Design review of the part built by this model. Coordinates are the model's own, in mm. Face numbers are marked on the shaded views. A direction names the side the tool comes from. Coordinates: 2 decimals unless noted, no trailing zeros. Loops run counter-clockwise (first coordinate to the right, second up) from the corner with the lowest first, then second, coordinate; pieces in that order, holes last. Notation, with made-up numbers: (54, 38) - (88, 38) arc R20 ccw to (88, 57) - close; hole circle Ø8 at (-0.75, -28). An arc over 180 degrees is marked (long way). Use one line per item in the form item = value. Start each with the question number.
(1) Clearance check with flat-ended pins moving along their axes: pin 1 Ø6 at (x, z) = (18, 10.5) entering from -Y; pin 2 Ø1.2 at (x, y) = (-1.5, 7.5) entering from +Z; pin 3 Ø2 at (x, y) = (15, 22) entering from +Z; pin 4 Ø2 at (x, z) = (-34, 3) entering from -Y. State where each tip first meets the part, or that it passes through.
(2) For L1, parallel to Z at x = 34, y = 3; L2, parallel to Z at x = 34, y = 8.75; L3, parallel to Y at x = 0, z = 1.15, list the stretches that pass through material, from the lowest coordinate up.
(3) Add section A-A (z = 3). State the section outline as (x, y) points, plus the area to 3 significant figures.
(4) Tool access review of the marked faces 5, 6 and 7: name each direction out of +Z, -Z, +X, -X, +Y, -Y from which nothing blocks a thin tool from reaching the whole face with its end or side.
(5) Add section D-D (x = 1). State the section outline as (y, z) points.
(6) Add section B-B (x = -28). State the section outline as (y, z) points.
(7) Add section C-C (y = 21.5). State the section outline as (x, z) points.
(8) The part is to be moulded in two halves that separate along Y. For the marked faces 1, 2, 3 and 4, say which applies: pulls with the +Y half, pulls with the -Y half, needs draft (parallel to the pull), parting line crosses it, or undercut.
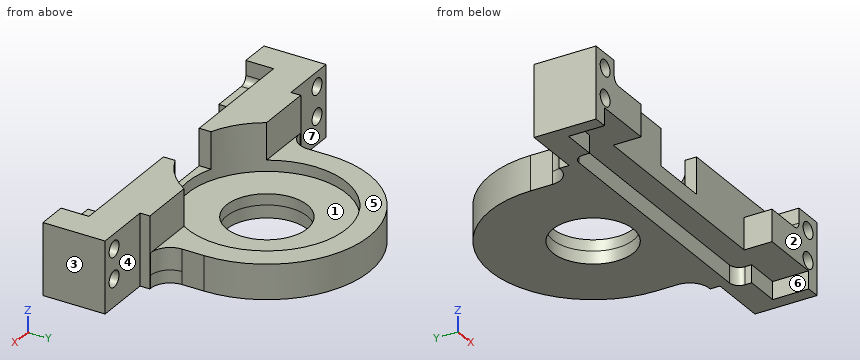
```python
from build123d import *

# Parameters (mm, degrees)
SKETCH2_R           = 16
BOSS_EXTRUDE1_DEPTH = 12
SKETCH3_R           = 16
SKETCH3_R_2         = 8.25
BOSS_EXTRUDE2_DEPTH = 2.5
CUT_EXTRUDE4_DEPTH  = 1
CUT_EXTRUDE5_REACH  = 60.683
SKETCH9_W           = 43.9
SKETCH9_H           = 5.7
SKETCH10_R          = 1.65
CUT_EXTRUDE6_DEPTH  = 59.87817932
CUT_EXTRUDE7_START  = -7.5
CUT_EXTRUDE7_DEPTH  = 7.5
FILETE1_R           = 2
FILETE2_R           = 4
SKETCH12_W          = 9
SKETCH12_H          = 5.7
CUT_EXTRUDE8_DEPTH  = 4.5
SKETCH15_W          = 12
SKETCH15_H          = 2.667603026
CUT_EXTRUDE10_DEPTH = 7.5
SKETCH16_R          = 8.25
BOSS_EXTRUDE3_DEPTH = 2.6
FILLET2_R           = 1.5
CUT_EXTRUDE11_REACH = 61.463
SKETCH17_W          = 11.722279144
SKETCH17_H          = 2
CUT_EXTRUDE12_START = -2.25
SKETCH18_R          = 16.25
CUT_EXTRUDE12_DEPTH = 9.75


with BuildPart() as part:
    # Sketch2 → Boss-Extrude1 (new body)
    with BuildSketch(Plane.XY):
        with BuildLine():
            Line((-21, 0), (21, 0))
            Line((21, 0), (37, 0))
            Line((37, 0), (37, 14.7))
            Line((37, 14.7), (21, 14.7))
            Line((21, 14.7), (21, 23.2))
            ThreePointArc((21, 23.2), (0, 44.2), (-21, 23.2))
            Line((-21, 23.2), (-21, 14.7))
            Line((-21, 14.7), (-37, 14.7))
            Line((-37, 14.7), (-37, 0))
            Line((-37, 0), (-21, 0))
        make_face()
        with Locations((0, 23.2)):
            Circle(SKETCH2_R, mode=Mode.SUBTRACT)
    extrude(amount=BOSS_EXTRUDE1_DEPTH)

    # Sketch3 → Boss-Extrude2 (add)
    with BuildSketch(Plane.XY):
        with Locations((0, 23.2)):
            Circle(SKETCH3_R)
        with Locations((0, 23.2)):
            Circle(SKETCH3_R_2, mode=Mode.SUBTRACT)
    extrude(amount=BOSS_EXTRUDE2_DEPTH)

    # Sketch8 → Cut-Extrude4 (cut)
    with BuildSketch(Plane.XY):
        Polygon((-27.15, 0), (27.15, 0), (34.2, 0), (34.2, 7.35), (27.15, 7.35), (27.15, 10.7), (-27.15, 10.7), (-27.15, 7.35), (-34.2, 7.35), (-34.2, 0), align=None)
    extrude(amount=CUT_EXTRUDE4_DEPTH, mode=Mode.SUBTRACT)

    # Sketch9 → Cut-Extrude5 (cut, up to next)
    with BuildSketch(Plane(origin=(0, 0, 1), x_dir=(-1, 0, 0), z_dir=(0, 0, -1)), mode=Mode.PRIVATE) as cut_extrude5_sk1:
        with Locations((0, 2.85)):
            Rectangle(SKETCH9_W, SKETCH9_H)
    cut_extrude5_tool1 = extrude(cut_extrude5_sk1.sketch, amount=-CUT_EXTRUDE5_REACH, mode=Mode.PRIVATE) & part.part
    add(cut_extrude5_tool1.solids().sort_by_distance((0, 2.85, 1))[0], mode=Mode.SUBTRACT)

    # Sketch10 → Cut-Extrude6 (cut, through all)
    with BuildSketch(Plane.XZ):
        with Locations((-34, 9)):
            Circle(SKETCH10_R)
        with Locations((-34, 3)):
            Circle(SKETCH10_R)
        with Locations((34, 3)):
            Circle(SKETCH10_R)
        with Locations((34, 9)):
            Circle(SKETCH10_R)
    extrude(amount=-CUT_EXTRUDE6_DEPTH, mode=Mode.SUBTRACT)

    # Sketch11 → Cut-Extrude7 (cut)
    with BuildSketch(Plane.XY.offset(12).offset(CUT_EXTRUDE7_START)):
        with BuildLine():
            Line((21, 14.7), (21, 23.2))
            ThreePointArc((21, 23.2), (0, 44.2), (-21, 23.2))
            Line((-21, 23.2), (-21, 14.7))
            Line((-21, 14.7), (21, 14.7))
        make_face()
    extrude(amount=CUT_EXTRUDE7_DEPTH, mode=Mode.SUBTRACT)

    # Filete1
    filete1_edges = [part.edges().sort_by_distance(p)[0] for p in [
        (27.15, 10.7, 0.5),
        (-27.15, 10.7, 0.5),
    ]]
    fillet(filete1_edges, radius=FILETE1_R)

    # Filete2
    filete2_edges = [part.edges().sort_by_distance(p)[0] for p in [
        (-21, 14.7, 2.25),
        (21, 14.7, 2.25),
    ]]
    fillet(filete2_edges, radius=FILETE2_R)

    # Sketch12 → Cut-Extrude8 (cut)
    with BuildSketch(Plane.XY.offset(12)):
        with Locations((26.45, 2.85)):
            Rectangle(SKETCH12_W, SKETCH12_H)
        with Locations((-26.45, 2.85)):
            Rectangle(SKETCH12_W, SKETCH12_H)
    extrude(amount=-CUT_EXTRUDE8_DEPTH, mode=Mode.SUBTRACT)

    # Sketch15 → Cut-Extrude10 (cut)
    with BuildSketch(Plane.XY.offset(12)):
        with Locations((0, 7.033801513)):
            Rectangle(SKETCH15_W, SKETCH15_H)
    extrude(amount=-CUT_EXTRUDE10_DEPTH, mode=Mode.SUBTRACT)

    # Sketch16 → Boss-Extrude3 (add)
    with BuildSketch(Plane(origin=(0, 0, 0), x_dir=(-1, 0, 0), z_dir=(0, 0, -1))):
        with BuildLine():
            Line((-37, 14.7), (-25, 14.7))
            ThreePointArc((-25, 14.7), (-22.171572875, 15.871572875), (-21, 18.7))
            Line((-21, 18.7), (-21, 23.2))
            ThreePointArc((-21, 23.2), (0, 44.2), (21, 23.2))
            Line((21, 23.2), (21, 18.7))
            ThreePointArc((21, 18.7), (22.171572875, 15.871572875), (25, 14.7))
            Line((25, 14.7), (37, 14.7))
            Line((37, 14.7), (37, 0))
            Line((37, 0), (34.2, 0))
            Line((34.2, 0), (34.2, 7.35))
            Line((34.2, 7.35), (27.15, 7.35))
            Line((27.15, 7.35), (27.15, 8.7))
            ThreePointArc((27.15, 8.7), (26.564213562, 10.114213562), (25.15, 10.7))
            Line((25.15, 10.7), (-25.15, 10.7))
            ThreePointArc((-25.15, 10.7), (-26.564213562, 10.114213562), (-27.15, 8.7))
            Line((-27.15, 8.7), (-27.15, 7.35))
            Line((-27.15, 7.35), (-34.2, 7.35))
            Line((-34.2, 7.35), (-34.2, 0))
            Line((-34.2, 0), (-37, 0))
            Line((-37, 0), (-37, 14.7))
        make_face()
        with Locations((0, 23.2)):
            Circle(SKETCH16_R, mode=Mode.SUBTRACT)
    extrude(amount=BOSS_EXTRUDE3_DEPTH)

    # Fillet2
    fillet2_edges = [part.edges().sort_by_distance(p)[0] for p in [
        (30.95, 2.85, 7.5),
        (-30.95, 2.85, 7.5),
    ]]
    fillet(fillet2_edges, radius=FILLET2_R)

    # Sketch17 → Cut-Extrude11 (cut, up to next)
    with BuildSketch(Plane.XY.offset(12), mode=Mode.PRIVATE) as cut_extrude11_sk1:
        with Locations((-31.138860428, 13.7)):
            Rectangle(SKETCH17_W, SKETCH17_H)
    cut_extrude11_tool1 = extrude(cut_extrude11_sk1.sketch, amount=-CUT_EXTRUDE11_REACH, mode=Mode.PRIVATE) & part.part
    # Sketch17 → Cut-Extrude11 (cut, up to next)
    with BuildSketch(Plane.XY.offset(12), mode=Mode.PRIVATE) as cut_extrude11_sk2:
        with Locations((31.138860428, 13.7)):
            Rectangle(SKETCH17_W, SKETCH17_H)
    cut_extrude11_tool2 = extrude(cut_extrude11_sk2.sketch, amount=-CUT_EXTRUDE11_REACH, mode=Mode.PRIVATE) & part.part
    add(cut_extrude11_tool1.solids().sort_by_distance((-31.13886, 13.7, 12))[0], mode=Mode.SUBTRACT)
    add(cut_extrude11_tool2.solids().sort_by_distance((31.13886, 13.7, 12))[0], mode=Mode.SUBTRACT)

    # Sketch18 → Cut-Extrude12 (cut)
    with BuildSketch(Plane.XY.offset(4.5).offset(CUT_EXTRUDE12_START)):
        with Locations((0, 23.2)):
            Circle(SKETCH18_R)
    extrude(amount=CUT_EXTRUDE12_DEPTH, mode=Mode.SUBTRACT)


solid = part.part
```
Computed values:
q1.pin_1 = 5.7
q1.pin_2 = 4.5
q1.pin_3 = 2.25
q1.pin_4 = through
q2.L1 = 1 to 1.35, 4.65 to 7.35, 10.65 to 12
q2.L2 = -2.6 to 1.35, 4.65 to 7.35, 10.65 to 12
q2.L3 = 5.7 to 14.95, 31.45 to 44.2
q3.outline = (-37, 0) - (-35.65, 0) - (-35.65, 12.7) - (-37, 12.7) - close; (-32.35, 0) - (-21.95, 0) - (-21.95, 5.7) - (21.95, 5.7) - (21.95, 0) - (32.35, 0) - (32.35, 12.7) - (25.28, 12.7) - (25.28, 14.7) - (25, 14.7) arc R4 cw to (21, 18.7) - (21, 23.2) arc R21 ccw to (-21, 23.2) - (-21, 18.7) arc R4 cw to (-25, 14.7) - (-25.28, 14.7) - (-25.28, 12.7) - (-32.35, 12.7) - close; (35.65, 0) - (37, 0) - (37, 12.7) - (35.65, 12.7) - close; hole circle Ø32.5 at (0, 23.2)
q3.area = 934 mm^2
q4.face_5 = +Z, +X, -X, +Y
q4.face_6 = -Z, -Y
q4.face_7 = +Z, -Z, -X, +Y
q5.outline = (5.7, 1) - (10.7, 1) - (10.7, -2.6) - (15.01, -2.6) - (15.01, 2.25) - (6.98, 2.25) - (6.98, 4.5) - (5.7, 4.5) - close; (31.39, -2.6) - (44.18, -2.6) - (44.18, 4.5) - (39.42, 4.5) - (39.42, 2.25) - (31.39, 2.25) - close
q6.outline = (0, 1) - (7.35, 1) - (7.35, -2.6) - (12.7, -2.6) - (12.7, 12) - (5.7, 12) - (5.7, 7.5) - (0, 7.5) - close
q7.outline = (-21, -2.6) - (-8.07, -2.6) - (-8.07, 2.25) - (-16.16, 2.25) - (-16.16, 4.5) - (-21, 4.5) - close; (8.07, -2.6) - (21, -2.6) - (21, 4.5) - (16.16, 4.5) - (16.16, 2.25) - (8.07, 2.25) - close
q8.face_1 = undercut
q8.face_2 = pulls with the -Y half
q8.face_3 = needs draft
q8.face_4 = pulls with the +Y half
